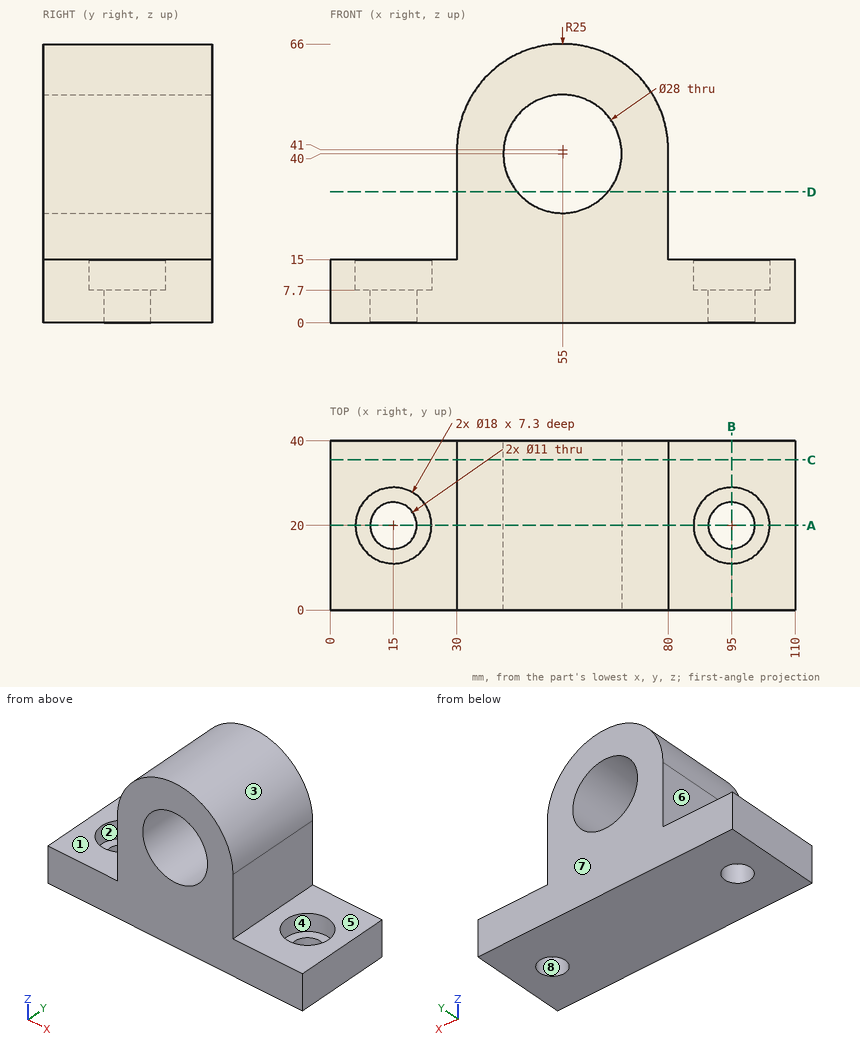
Part print with two shaded views. Sizes in mm from the minimum x, y, z corner. A direction names the side the tool comes from. Give positions to 0.01 mm unless a question says otherwise; leave off trailing zeros. Order: outer loops, then holes, each group sorted by start corner. A loop starts at its lowest first (then second) coordinate and runs counter-clockwise, first axis right, second up.
1) Saw through at C-C, the plane y = 35.5. Write the cut outline in (x, z), then the cut area to 3 significant figures.
2) Pin check, flat tips, straight feed: pin 1 (21 mm diameter, centred on y = 19.5, z = 33, fed in from -X); pin 2 (1.5 mm diameter, centred on x = 68, y = 33, fed in from +Z); pin 3 (9 mm diameter, centred on x = 95.5, y = 18, fed in from +Z); pin 4 (25 mm diameter, centred on x = 55, z = 40, fed in from -Y). Stop position of each tip, or through.
3) Mould opens along X. For the marked faces 1, 2 and 3 say: +X half, -X half, draft (parallel to the pull), parting line (faces both ways), or undercut.
4) Wall check: probe 1 along Y at (x, z) = (95, 10); probe 2 along Z at (x, y) = (14, 6); probe 3 along Z at (x, y) = (45, 12.5). Give the ranges that are in metal, low to high.
5) 3-axis set-ups, long thin cutter, end or side, ignore diameter. For the marked faces 4, 5, 6, 7 and 8: which of +Z, -Z, +X, -X, +Y, -Y reach the whole face in a straight line?
6) Saw through at D-D, the plane z = 31. Write the cut outline in (x, y), then the cut area to 3 significant figures.
7) Saw through at A-A, the plane y = 20. Write the cut outline in (x, z), then the cut area to 3 significant figures.
8) Saw through at B-B, the plane x = 95. Write the cut outline in (y, z), then the cut area to 3 significant figures.
Computed:
1. outline: (0, 0) - (110, 0) - (110, 15) - (80, 15) - (80, 41) arc R25 ccw to (30, 41) - (30, 15) - (0, 15) - close; hole circle Ø28 at (55, 40)
1. area: 3,320 mm2
2. pin 1: stops at x = 30
2. pin 2: stops at z = 62.79
2. pin 3: stops at z = 7.7
2. pin 4: passes through
3. face 1: draft
3. face 2: undercut
3. face 3: parting line
4. probe 1: y = 0 to 11, 29 to 40
4. probe 2: z = 0 to 15
4. probe 3: z = 0 to 30.2, 49.8 to 63.91
5. face 4: +Z
5. face 5: +Z, +X, +Y, -Y
5. face 6: +Z, -X, +Y, -Y
5. face 7: +Z, -Z, +X, -X, +Y
5. face 8: +Z, -Z
6. outline: (30, 0) - (44.28, 0) - (44.28, 40) - (30, 40) - close; (65.72, 0) - (80, 0) - (80, 40) - (65.72, 40) - close
6. area: 1,140 mm2
7. outline: (0, 0) - (9.5, 0) - (9.5, 7.7) - (6, 7.7) - (6, 15) - (0, 15) - close; (20.5, 0) - (89.5, 0) - (89.5, 7.7) - (86, 7.7) - (86, 15) - (80, 15) - (80, 41) arc R25 ccw to (30, 41) - (30, 15) - (24, 15) - (24, 7.7) - (20.5, 7.7) - close; (100.5, 0) - (110, 0) - (110, 15) - (104, 15) - (104, 7.7) - (100.5, 7.7) - close; hole circle Ø28 at (55, 40)
7. area: 2,880 mm2
8. outline: (0, 0) - (14.5, 0) - (14.5, 7.7) - (11, 7.7) - (11, 15) - (0, 15) - close; (25.5, 0) - (40, 0) - (40, 15) - (29, 15) - (29, 7.7) - (25.5, 7.7) - close
8. area: 384 mm2
